Verification items for this drawing (mm, ordinates from the low corner). Give positions to 0.01 mm unless a question says otherwise; leave off trailing zeros. Loops run counter-clockwise (first coordinate to the right, second up) from the corner with the lowest first, then second, coordinate; pieces in that order, holes last. Notation, with made-up numbers: M -26,-23 L -10,-23 A7 cw -10,-10 Z; hole C 35.5,-5 d6. An arc over 180 degrees is marked long. Use a Markdown table: item, result.
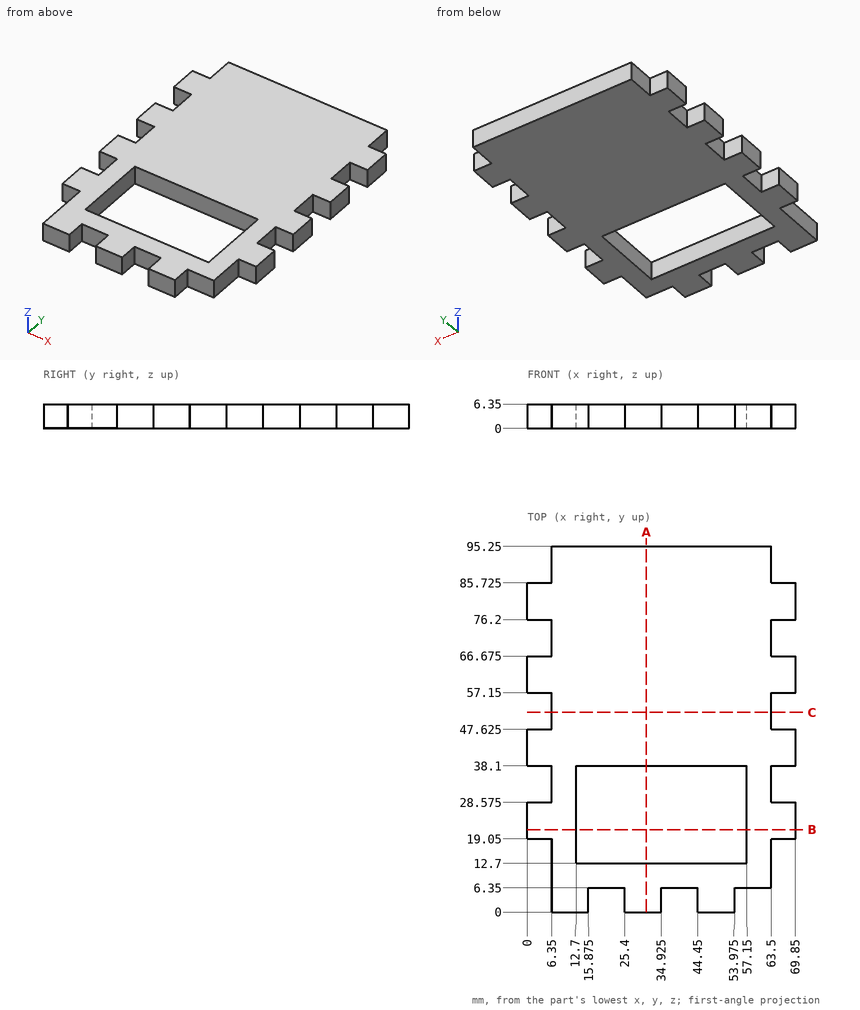
(1) Cross-section at A-A on x = 31. Record the cut outline in (y, z).
Results below:
| item | result |
|---|---|
| outline | M 0,0 L 12.7,0 L 12.7,6.35 L 0,6.35 Z; M 38.1,0 L 95.25,0 L 95.25,6.35 L 38.1,6.35 Z |
(2) Gauge pin test, flat ends, axial feed: P1, Ø1.9, axis at y = 35, z = 4, coming from the -X side; P2, Ø3, axis at x = 65.5, z = 4, coming from the -Y side; P3, Ø1.9, axis at x = 3, z = 4, coming from the +Y side (3 decimals). Record the tip position at first contact, or that the pin passes through.
Results below:
| item | result |
|---|---|
| P1 | x = 6.35 |
| P2 | y = 19.05 |
| P3 | y = 85.725 |
(3) Material ranges on line 1 (X direction, y = 4.5, z = 3.25) (3 decimals); line 2 (Y direction, x = 20.5, z = 1.75); line 3 (Y direction, x = 14, z = 0.5), recorded low to high.
Results below:
| item | result |
|---|---|
| line 1 | 6.35 to 15.875, 25.4 to 34.925, 44.45 to 53.975 |
| line 2 | 6.35 to 12.7, 38.1 to 95.25 |
| line 3 | 0 to 12.7, 38.1 to 95.25 |
(4) Cross-section at C-C on y = 52. Record the cut outline in (x, z), then the cut area to 3 significant figures.
Results below:
| item | result |
|---|---|
| outline | M 6.35,0 L 63.5,0 L 63.5,6.35 L 6.35,6.35 Z |
| area | 363 mm^2 |
(5) Cross-section at B-B on y = 21.5. Record the cut outline in (x, z), then the cut area to 3 significant figures.
Results below:
| item | result |
|---|---|
| outline | M 0,0 L 12.7,0 L 12.7,6.35 L 0,6.35 Z; M 57.15,0 L 69.85,0 L 69.85,6.35 L 57.15,6.35 Z |
| area | 161 mm^2 |
